For this review, take the finished solid that the model builds, in its own axes (mm). Face numbers are marked on the shaded views. A direction names the side the tool comes from. Give positions to 0.01 mm unless a question says otherwise; leave off trailing zeros. Write each loop counter-clockwise with the first axis right and the second up, starting at its lowest first coordinate (ties: lowest second). Pieces come first, ordered by that corner, then holes. Notation, with made-up numbers: M -11,59 L 24,59 A7 ccw 24,66 Z; hole C 66.25,63 d9. An arc over 180 degrees is marked long. Use one line per item in the form item = value. Start each with the question number.
Q1. Consider section B-B on x = 50. Write out the cut boundary in (y, z).
Q2. Clearance check with flat-ended pins moving along their axes: pin 1 Ø6 at (y, z) = (22, -15) entering from +X; pin 2 Ø21 at (x, y) = (0, 54) entering from -Z; pin 3 Ø1 at (x, z) = (20.5, 18.5) entering from +Y. State where each tip first meets the part, or that it passes through.
Q3. Consider section C-C on y = 26.5. Write out the cut boundary in (x, z), and give its area (3 significant figures).
Q4. Mouldability with a two-part tool opening along Y and no side actions: class the marked faces 1, 2 and 3 as released by +Y, released by -Y, zero draft, split by the parting line, or undercut.
Q5. Consider section A-A on x = 0. Write out the cut boundary in (y, z), and give its area (3 significant figures).
Q6. Tool access review of the marked faces 4, 5 and 6: name each direction out of +Z, -Z, +X, -X, +Y, -Y from which nothing blocks a thin tool from reaching the whole face with its end or side.
Q7. For probe 1 along Z at (x, y) = (10, 55); probe 2 along Y at (x, z) = (0, 20.75); probe 3 along Y at (x, z) = (23, -12), list the stretches that pass through material, from the lowest coordinate up. Write a range as [from, to].
Q8. Consider section D-D on z = 0. Write out the cut boundary in (x, y).
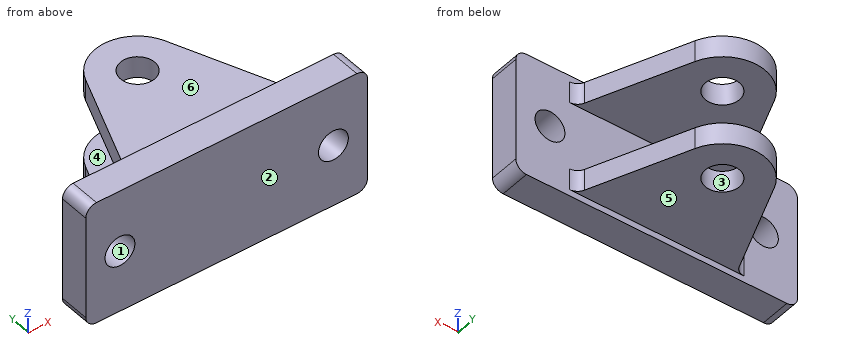
```python
from build123d import *

# Parameters (mm, degrees)
SKETCH1_W           = 132
SKETCH1_H           = 58
BOSS_EXTRUDE1_DEPTH = 14.167595312
SKETCH2_R           = 7
CUT_EXTRUDE1_DEPTH  = 74.469182362
BOSS_EXTRUDE2_START = 16
BOSS_EXTRUDE2_DEPTH = 10
CUT_EXTRUDE2_REACH  = 115.389
SKETCH4_R           = 8
BOSS_EXTRUDE3_START = -26
BOSS_EXTRUDE3_DEPTH = 10
CUT_EXTRUDE3_REACH  = 115.389
SKETCH5_R           = 8
FILLET1_R           = 5


with BuildPart() as part:
    # Sketch1 → Boss-Extrude1 (new body)
    with BuildSketch(Plane(origin=(0, 0, 0), x_dir=(1, 0, 0), z_dir=(0, 1, 0))):
        Rectangle(SKETCH1_W, SKETCH1_H)
    extrude(amount=BOSS_EXTRUDE1_DEPTH)

    # Sketch2 → Cut-Extrude1 (cut, through all)
    with BuildSketch(Plane(origin=(0, 14.167595312, 0), x_dir=(1, 0, 0), z_dir=(0, 1, 0))):
        with Locations(Location((-50, 0, 0), (0, 0, 270))):
            Circle(SKETCH2_R)
        with Locations(Location((50, 0, 0), (0, 0, 90))):
            Circle(SKETCH2_R)
    extrude(amount=-CUT_EXTRUDE1_DEPTH, mode=Mode.SUBTRACT)

    # Sketch3 → Boss-Extrude2 (add)
    with BuildSketch(Plane.XY.offset(BOSS_EXTRUDE2_START)):
        with BuildLine():
            Line((37.5, 14.167595312), (-37.5, 14.167595312))
            Line((-37.5, 14.167595312), (-18.565958618, 61.436745296))
            ThreePointArc((-18.565958618, 61.436745296), (0, 74), (18.565958618, 61.436745296))
            Line((18.565958618, 61.436745296), (37.5, 14.167595312))
        make_face()
    extrude(amount=BOSS_EXTRUDE2_DEPTH)

    # Sketch4 → Cut-Extrude2 (cut, up to next)
    with BuildSketch(Plane.XY.offset(26), mode=Mode.PRIVATE) as cut_extrude2_sk1:
        with Locations((0, 54)):
            Circle(SKETCH4_R)
    cut_extrude2_tool1 = extrude(cut_extrude2_sk1.sketch, amount=-CUT_EXTRUDE2_REACH, mode=Mode.PRIVATE) & part.part
    add(cut_extrude2_tool1.solids().sort_by_distance((0, 54, 26))[0], mode=Mode.SUBTRACT)

    # Sketch3_2 → Boss-Extrude3 (add)
    with BuildSketch(Plane.XY.offset(BOSS_EXTRUDE3_START)):
        with BuildLine():
            Line((37.5, 14.167595312), (-37.5, 14.167595312))
            Line((-37.5, 14.167595312), (-18.565958618, 61.436745296))
            ThreePointArc((-18.565958618, 61.436745296), (0, 74), (18.565958618, 61.436745296))
            Line((18.565958618, 61.436745296), (37.5, 14.167595312))
        make_face()
    extrude(amount=BOSS_EXTRUDE3_DEPTH)

    # Sketch5 → Cut-Extrude3 (cut, up to next)
    with BuildSketch(Plane(origin=(0, 0, -26), x_dir=(-1, 0, 0), z_dir=(0, 0, -1)), mode=Mode.PRIVATE) as cut_extrude3_sk1:
        with Locations(Location((0, 54, 0), (0, 0, 180))):
            Circle(SKETCH5_R)
    cut_extrude3_tool1 = extrude(cut_extrude3_sk1.sketch, amount=-CUT_EXTRUDE3_REACH, mode=Mode.PRIVATE) & part.part
    add(cut_extrude3_tool1.solids().sort_by_distance((0, 54, -26))[0], mode=Mode.SUBTRACT)

    # Fillet1
    fillet1_edges = [part.edges().sort_by_distance(p)[0] for p in [
        (37.5, 14.167595312, 21),
        (-37.5, 14.167595312, 21),
        (37.5, 14.167595312, -21),
        (-37.5, 14.167595312, -21),
        (-66, 7.083797656, 29),
        (66, 7.083797656, 29),
        (66, 7.083797656, -29),
        (-66, 7.083797656, -29),
    ]]
    fillet(fillet1_edges, radius=FILLET1_R)


solid = part.part
```
Working result:
q1.outline = M 0,-29 L 14.17,-29 L 14.17,-7 L 0,-7 Z; M 0,7 L 14.17,7 L 14.17,29 L 0,29 Z
q2.pin_1 = 35.5
q2.pin_2 = -26
q2.pin_3 = 57.86
q3.outline = M -32.56,-26 L 32.56,-26 L 32.56,-16 L -32.56,-16 Z; M -32.56,16 L 32.56,16 L 32.56,26 L -32.56,26 Z
q3.area = 1,300 mm²
q4.face_1 = zero draft
q4.face_2 = released by -Y
q4.face_3 = undercut
q5.outline = M 0,-29 L 14.17,-29 L 14.17,-26 L 46,-26 L 46,-16 L 14.17,-16 L 14.17,16 L 46,16 L 46,26 L 14.17,26 L 14.17,29 L 0,29 Z; M 62,-26 L 74,-26 L 74,-16 L 62,-16 Z; M 62,16 L 74,16 L 74,26 L 62,26 Z
q5.area = 1,700 mm²
q6.face_4 = +X, -X, +Y
q6.face_5 = -Z, +X, -X, +Y
q6.face_6 = +Z, +X, -X, +Y
q7.probe_1 = [-26, -16], [16, 26]
q7.probe_2 = [0, 46], [62, 74]
q7.probe_3 = [0, 14.17]
q8.outline = M -66,0 L -57,0 L -57,14.17 L -66,14.17 Z; M -43,0 L 43,0 L 43,14.17 L -43,14.17 Z; M 57,0 L 66,0 L 66,14.17 L 57,14.17 Z
